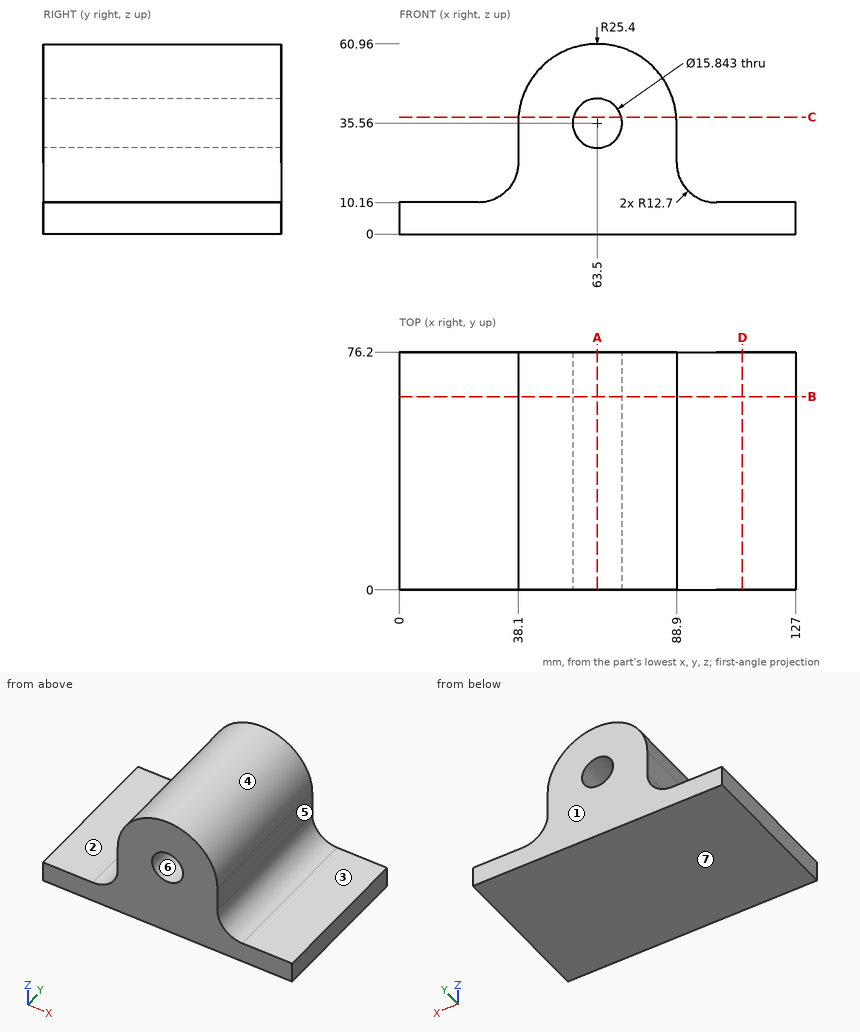
Answer from the drawing. Dimensions are ordinates in mm from the lowest x, y and z of the part. A direction names the side the tool comes from. Coordinates: 2 decimals unless noted, no trailing zeros. Write each loop counter-clockwise with the first axis right and the second up, starting at its lowest first coordinate (ties: lowest second). Pieces come first, ordered by that corner, then holes. Notation, with made-up numbers: (56.5, 14.5) - (67.5, 14.5) arc R23 cw to (67.5, 26.5) - close; hole circle Ø5 at (-36.75, 21.5). An arc over 180 degrees is marked (long way). One line per question, with ' | ' between items.
Q1. Find section A-A, the plane x = 63.5. Write down the section's boundary in (y, z).
Result set:
outline: (0, 0) - (76.2, 0) - (76.2, 27.64) - (0, 27.64) - close; (0, 43.48) - (76.2, 43.48) - (76.2, 60.96) - (0, 60.96) - close
Q2. Determine the mould class of the marked faces 4, 5, 6 and 7 for opening direction X: +X half, -X half, draft (parallel to the pull), parting line (faces both ways), or undercut.
Result set:
face 4: parting line | face 5: +X half | face 6: undercut | face 7: draft
Q3. Each of these flat-tipped pins is pushed along its axis until it touches: P1, Ø4, axis at y = 48, z = 30.5, coming from the -X side; P2, Ø6.5, axis at y = 36.5, z = 27.5, coming from the +X side; P3, Ø7.5, axis at x = 14, y = 37, coming from the +Z side; P4, Ø12, axis at x = 55.5, y = 24, coming from the -Z side. Where does it stop, or does it pass through?
Result set:
P1: x = 38.1 | P2: x = 88.9 | P3: z = 10.16 | P4: z = 0
Q4. Find section D-D, the plane x = 110. Write down the section's boundary in (y, z), plus the area to 3 significant figures.
Result set:
outline: (0, 0) - (76.2, 0) - (76.2, 10.16) - (0, 10.16) - close | area: 774 mm^2
Q5. Consider L1, parallel to X at y = 55, z = 35; L2, parallel to Z at x = 63.5, y = 17; L3, parallel to Z at x = 63, y = 29 (1 decimal). Determine where each line is inside the solid, lowest interval first. Write a range as [from, to].
Result set:
L1: [38.1, 55.6], [71.4, 88.9] | L2: [0, 27.64], [43.48, 60.96] | L3: [0, 27.7], [43.5, 61]
Q6. Find section C-C, the plane z = 37.5. Write down the section's boundary in (x, y) (1 decimal).
Result set:
outline: (38.2, 0) - (55.8, 0) - (55.8, 76.2) - (38.2, 76.2) - close; (71.2, 0) - (88.8, 0) - (88.8, 76.2) - (71.2, 76.2) - close
Q7. Find section B-B, the plane y = 62. Write down the section's boundary in (x, z).
Result set:
outline: (0, 0) - (127, 0) - (127, 10.16) - (101.6, 10.16) arc R12.7 cw to (88.9, 22.86) - (88.9, 35.56) arc R25.4 ccw to (38.1, 35.56) - (38.1, 22.86) arc R12.7 cw to (25.4, 10.16) - (0, 10.16) - close; hole circle Ø15.84 at (63.5, 35.56)
Q8. For the marked faces 1, 2 and 3, determine the directions among +Z, -Z, +X, -X, +Y, -Y from which every point of the face is accessible in a straight line to the end or side of a thin tool.
Result set:
face 1: +Z, -Z, +X, -X, +Y | face 2: +Z, -X, +Y, -Y | face 3: +Z, +X, +Y, -Y
